The model under review builds one solid part; all positions refer to its coordinate system, in mm. Face numbers are marked on the shaded views. A direction names the side the tool comes from. Round coordinates to 2 decimals unless told otherwise and drop trailing zeros. Write each loop counter-clockwise with the first axis right and the second up, starting at its lowest first coordinate (ties: lowest second). Pieces come first, ordered by that corner, then holes. Notation, with made-up numbers: M 1,-25 L 9,-25 A19 cw 9,8 Z; hole C 44.5,17 d4. An arc over 180 degrees is marked long. Write item = value, one per line. Start each with the question number.
Item 1: Take a section at C-C, the plane z = 4. Give the boundary of the cut face in (x, y), plus the area to 3 significant figures.
Item 2: The part is to be moulded in two halves that separate along Z. For the marked faces 3, 4 and 5, say which applies: +Z half, -Z half, draft (parallel to the pull), parting line (faces both ways), or undercut.
Item 3: Take a section at B-B, the plane x = 0. Give the boundary of the cut face in (y, z), plus the area to 3 significant figures.
Item 4: Take a section at A-A, the plane y = 7. Give the number of separate pieces and of enclosed holes in the cut face, plus the area to 3 significant figures.
Item 5: Tool access review of the marked faces 1 and 2: name each direction out of +Z, -Z, +X, -X, +Y, -Y from which nothing blocks a thin tool from reaching the whole face with its end or side.
Item 6: To check wall thickness, follow line 1 along Z through (x, y) = (15, 0.8); line 2 along X through (y, z) = (3, 15). State the ranges of each line that lie inside material, in increasing order.
Item 7: For pin 1 Ø4 at (x, z) = (-15, 15) entering from +Y; pin 2 Ø4 at (x, y) = (2, 1) entering from -Z; pin 3 Ø1 at (x, y) = (-0.5, 6) entering from +Z, all flat-tipped, find the tip position at first contact; note any pin that passes through.
Autodesk Fusion 360 part; units mm, degrees
sketch "Skizze1" plane through (0, 0, 0) normal (0, 1, 0) x (1, 0, 0)
  line L0 (-26.0309, 15.2828) -> (-26.0309, -15.2828)
  line L1 (-26.0309, -15.2828) -> (-15.2828, -26.0309)
  line L2 (-15.2828, -26.0309) -> (15.2828, -26.0309)
  line L3 (15.2828, -26.0309) -> (26.0309, -15.2828)
  line L4 (26.0309, -15.2828) -> (26.0309, 15.2828)
  line L5 (26.0309, 15.2828) -> (15.2828, 26.0309)
  line L6 (15.2828, 26.0309) -> (-15.2828, 26.0309)
  line L7 (-15.2828, 26.0309) -> (-26.0309, 15.2828)
  circle A0 centre (-15, 15) radius 1.65
  line L8 (0, 26.0309) -> (0, -26.0309) construction
  line L9 (-26.0309, 0) -> (26.0309, 0) construction
  circle A1 centre (15, 15) radius 1.65
  circle A2 centre (15, -15) radius 1.65
  circle A3 centre (-15, -15) radius 1.65
  line L10 (-26.0309, 15.2828) -> (-10.748, 0)
  line L11 (-10.748, 0) -> (-26.0309, -15.2828)
  line L12 (-15.2828, 26.0309) -> (0, 10.748)
  line L13 (0, 10.748) -> (15.2828, 26.0309)
  line L14 (26.0309, 15.2828) -> (10.748, 0)
  line L15 (10.748, 0) -> (26.0309, -15.2828)
  line L16 (15.2828, -26.0309) -> (0, -10.748)
  line L17 (-15.2828, -26.0309) -> (0, -10.748)
  arc A4 (-26.0309, -13.2828) -> (-26.0309, 13.2828) centre (-40.983, 0) ccw
  arc A5 (13.2828, -26.0309) -> (-13.2828, -26.0309) centre (0, -40.983) ccw
  arc A6 (26.0309, 13.2828) -> (26.0309, -13.2828) centre (40.983, 0) ccw
  arc A7 (-13.2828, 26.0309) -> (13.2828, 26.0309) centre (0, 40.983) ccw
  dimension "d1" = 15.2
  dimension "d2" = 3.3
  dimension "d3" = 8
  dimension "d4" = 15
  dimension "d5" = 15
  dimension "d6" = 45
  dimension "d7" = 2
  dimension "d8" = 2
  dimension "d10" = 20
  dimension "d12" = 360
extrude "Extrusion1" add sketch "Skizze1" along normal blind 1.5 contours L0 L10 L11 A4 | L1 L3 L5 L7 L10 L11 L12 L13 L14 L15 L16 L17 | L6 L12 L13 A7 | L2 L16 L17 A5 | L4 L14 L15 A6
extrude "Extrusion2" add sketch "Skizze1" along normal blind 8 contours L0 L10 L11 A4 | L6 L12 L13 A7 | L2 L16 L17 A5 | L4 L14 L15 A6
fillet "Abrundung1" radius 1.5 4 edges at (0, 4.75, -10.748) (10.748, 4.75, 0) (0, 4.75, 10.748) (-10.748, 4.75, 0)
fillet "Abrundung3" radius 2 8 edges at (-26.0309, 4, 13.2828) (-26.0309, 4, -13.2828) (-13.2828, 4, 26.0309) (13.2828, 4, 26.0309) (26.0309, 4, 13.2828) (26.0309, 4, -13.2828) (13.2828, 4, -26.0309) (-13.2828, 4, -26.0309)
equation "d8 = d7"
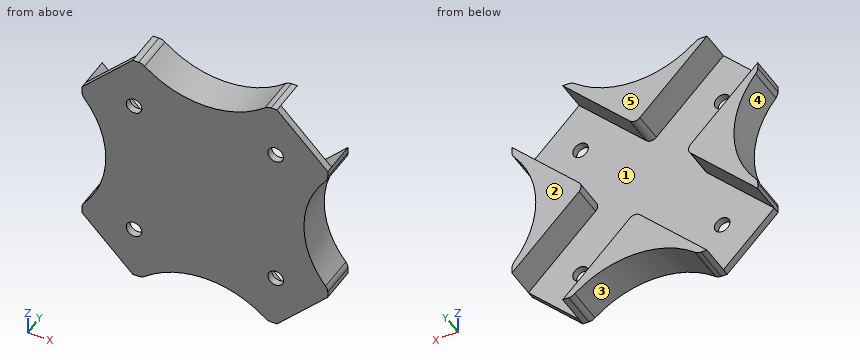
Response values:
q1.outline = M -21.39,0 L 21.39,0 L 21.39,8 L 14.75,8 L 14.75,1.5 L -14.75,1.5 L -14.75,8 L -21.39,8 Z
q1.area = 150 mm2
q2.face_3 = -Z half
q2.face_4 = undercut
q2.face_5 = draft
q3.outline = M 0,-20.98 L 8,-20.98 L 8,-11.37 L 1.5,-11.37 L 1.5,11.37 L 8,11.37 L 8,20.98 L 0,20.98 Z
q3.area = 188 mm2
q4.separate_pieces = 4
q4.enclosed_holes = 0
q4.area = 564 mm2
q5.face_1 = +Y
q5.face_2 = +Z, -Z, +X, -X, +Y
q6.line_1 = -26.03 to -16.65, -13.35 to 13.35, 16.65 to 26.03
q6.line_2 = -26.03 to -25.75, -4.25 to 4.25, 25.75 to 26.03
q7.pin_1 = 1.5
q7.pin_2 = -21.39
q7.pin_3 = 21.01
